Source: CAD feature listing. Evaluate the final solid. Frame: model axes, mm. A direction names the side the tool comes from. Give positions to 0.01 mm unless a question says otherwise; leave off trailing zeros. Order: outer loops, then holes, each group sorted by start corner. A loop starts at its lowest first (then second) coordinate and runs counter-clockwise, first axis right, second up.
1) Material intervals for line 1 (X direction, y = 30, z = 5); line 2 (Y direction, x = 0, z = 21.9), sorted ascending.
2) First-contact query: P1, Ø3.5, axis at x = 0, y = 0, coming from the +Z side. Flat tip, straight axial feed; report the tip coordinate or a pass-through.
3) Access query for faces 4 (the face through (-36.5, -1, 10)), 5 (the face through (-13.72, 18.76, 22.46)), 6 (the face through (-1, -41.5, 12)). Directions: +Z, -Z, +X, -X, +Y, -Y. A direction counts if a zero-diameter tool reaches every point of the face in a straight line with its end or side. Return the directions, or none.
4) Draft query along X for faces 1 (the face through (9.197, 34.705, 22.465)), 2 (the face through (25.457, -25.318, 22.465)), 3 (the face through (-1, 41.5, 12)). Return one class per face: released by +X, released by -X, zero draft, split by the parting line, or undercut.
5) Section B-B, the plane z = 17.5. Return loops of the section in (x, y), plus the area to 3 significant figures.
6) Section A-A, the plane y = 0. Return loops of the section in (x, z), plus the area to 3 significant figures.
7) Section D-D, the plane y = -25. Return loops of the section in (x, z) (1 decimal), plus the area to 3 significant figures.
```python
from build123d import *

# Parameters (mm, degrees)
F0_W     = 83
F0_H     = 83
F0_W_2   = 73
F0_H_2   = 73
F1_DEPTH = 20
F4_DEPTH = 10
F5_W     = 83
F5_H     = 83
F5_R     = 1.5
F6_DEPTH = 5
F7_R     = 2


with BuildPart() as f1:
    # F0 (on Top) → F1 (new body)
    with BuildSketch(Plane.XY):
        Rectangle(F0_W, F0_H)
        Rectangle(F0_W_2, F0_H_2, mode=Mode.SUBTRACT)
    extrude(amount=F1_DEPTH)

    # F2: F1 across plane


with BuildPart() as f1_1:
    add(f1.part)
    add(f1.part.mirror(Plane.YZ))

    # F3 (on face) → F4 (cut)
    with BuildSketch(Plane(origin=(0, 0, 0), x_dir=(1, 0, 0), z_dir=(0, 0, -1))):
        Polygon((36.5, 32), (39, 32), (39, 39), (32, 39), (32, 36.5), (36.5, 36.5), align=None)
        Polygon((-39, -32), (-39, -39), (-32, -39), (-32, -36.5), (-36.5, -36.5), (-36.5, -32), align=None)
    extrude(amount=-F4_DEPTH, mode=Mode.SUBTRACT)

    # F5 (on face) → F6 (join)
    with BuildSketch(Plane.XY.offset(20)):
        Rectangle(F5_W, F5_H)
        Polygon((36.5, 2.5), (36.5, -2.5), (36.5, -36.5), (2.5, -36.5), (-2.5, -36.5), (-36.5, -36.5), (-36.5, -2.5), (-36.5, 2.5), (-36.5, 36.5), (-2.5, 36.5), (2.5, 36.5), (36.5, 36.5), align=None, mode=Mode.SUBTRACT)
        Polygon((36.5, -36.5), (36.5, -2.5), (36.5, 2.5), (36.5, 36.5), (2.5, 36.5), (-2.5, 36.5), (-36.5, 36.5), (-36.5, 2.5), (-36.5, -2.5), (-36.5, -36.5), (-2.5, -36.5), (2.5, -36.5), align=None)
        Polygon((-2.5, -9.3301270189), (-2.5, -36.5), (-16.0849364905, -32.8599272381), align=None, mode=Mode.SUBTRACT)
        Polygon((-32.8599272381, -16.0849364905), (-36.5, -2.5), (-9.3301270189, -2.5), align=None, mode=Mode.SUBTRACT)
        Polygon((-6.8301270189, -6.8301270189), (-20.4150635095, -30.3599272381), (-30.3599272381, -20.4150635095), align=None, mode=Mode.SUBTRACT)
        Polygon((16.0849364905, -32.8599272381), (2.5, -36.5), (2.5, -9.3301270189), align=None, mode=Mode.SUBTRACT)
        Polygon((6.8301270189, -6.8301270189), (30.3599272381, -20.4150635095), (20.4150635095, -30.3599272381), align=None, mode=Mode.SUBTRACT)
        Polygon((9.3301270189, -2.5), (36.5, -2.5), (32.8599272381, -16.0849364905), align=None, mode=Mode.SUBTRACT)
        Polygon((-9.3301270189, 2.5), (-36.5, 2.5), (-32.8599272381, 16.0849364905), align=None, mode=Mode.SUBTRACT)
        Polygon((-30.3599272381, 20.4150635095), (-20.4150635095, 30.3599272381), (-6.8301270189, 6.8301270189), align=None, mode=Mode.SUBTRACT)
        Polygon((-16.0849364905, 32.8599272381), (-2.5, 36.5), (-2.5, 9.3301270189), align=None, mode=Mode.SUBTRACT)
        Circle(F5_R, mode=Mode.SUBTRACT)
        Polygon((20.4150635095, 30.3599272381), (30.3599272381, 20.4150635095), (6.8301270189, 6.8301270189), align=None, mode=Mode.SUBTRACT)
        Polygon((32.8599272381, 16.0849364905), (36.5, 2.5), (9.3301270189, 2.5), align=None, mode=Mode.SUBTRACT)
        Polygon((2.5, 9.3301270189), (2.5, 36.5), (16.0849364905, 32.8599272381), align=None, mode=Mode.SUBTRACT)
    extrude(amount=F6_DEPTH)

    # F7
    f7_edges = [f1_1.edges().sort_by_distance(p)[0] for p in [
        (-1.5, 0, 25),
    ]]
    fillet(f7_edges, radius=F7_R)


solid = f1_1.part
```
From the geometry:
1. line 1: x = -41.5 to -36.5, 36.5 to 41.5
1. line 2: y = -41.5 to -1.5, 1.5 to 41.5
2. P1: stops at z = 23.97
3. face 4: -Z
3. face 5: +Z, -Z
3. face 6: +Z, -Z, +X, -X, -Y
4. face 1: undercut
4. face 2: undercut
4. face 3: zero draft
5. outline: (-41.5, -41.5) - (41.5, -41.5) - (41.5, 41.5) - (-41.5, 41.5) - close; hole (-36.5, -36.5) - (36.5, -36.5) - (36.5, 36.5) - (-36.5, 36.5) - close
5. area: 1,560 mm2
6. outline: (-41.5, 0) - (-36.5, 0) - (-36.5, 20) - (-1.5, 20) - (-1.5, 23) arc R2 ccw to (-3.5, 25) - (-41.5, 25) - close; (1.5, 20) - (36.5, 20) - (36.5, 0) - (41.5, 0) - (41.5, 25) - (3.5, 25) arc R2 ccw to (1.5, 23) - close
6. area: 598 mm2
7. outline: (-41.5, 0) - (-36.5, 0) - (-36.5, 20) - (-25.8, 20) - (-25.8, 25) - (-41.5, 25) - close; (-17.3, 20) - (-11.5, 20) - (-11.5, 25) - (-17.3, 25) - close; (-2.5, 20) - (2.5, 20) - (2.5, 25) - (-2.5, 25) - close; (11.5, 20) - (17.3, 20) - (17.3, 25) - (11.5, 25) - close; (25.8, 20) - (36.5, 20) - (36.5, 0) - (41.5, 0) - (41.5, 25) - (25.8, 25) - close
7. area: 440 mm2
